from build123d import *

# Parameters (mm, degrees)
SKETCH004_W   = 113.720292
SKETCH004_H   = 7.903844
SKETCH004_R   = 1.75
SKETCH004_R_2 = 1.5
PAD_DEPTH     = 1


with BuildPart() as part:
    # Sketch004 → Pad (new body)
    with BuildSketch(Plane.XY):
        Rectangle(SKETCH004_W, SKETCH004_H)
        with Locations((-52.5, 0)):
            Circle(SKETCH004_R, mode=Mode.SUBTRACT)
        with Locations((52.5, 0)):
            Circle(SKETCH004_R, mode=Mode.SUBTRACT)
        Circle(SKETCH004_R_2, mode=Mode.SUBTRACT)
    extrude(amount=PAD_DEPTH)


solid = part.part
Verification items for the finished model (mm, model axes). Coordinates: 2 decimals unless noted, no trailing zeros. Order: outer loops, then holes, each group sorted by start corner. A loop starts at its lowest first (then second) coordinate and runs counter-clockwise, first axis right, second up. Notation, with made-up numbers: (-4.5, -14) -> (49.5, -14) arc R30 cw to (49.5, 12) -> close; hole circle Ø2 at (85.5, 63.5). An arc over 180 degrees is marked (long way). Put each result on its own line as item: value. Start each with the question number.
1. Material ranges on L1, parallel to Y at x = -52.5, z = 0.3; L2, parallel to Y at x = 1, z = 0.1, recorded low to high. Write a range as [from, to].
2. Go/stop test with flat-tipped pins: pin 1 Ø2 at (x, y) = (52.5, 0) entering from +Z; pin 2 Ø4 at (x, y) = (0, -1.5) entering from -Z. Record where each tip stops, or that it passes through.
3. Cross-section at C-C, the plane z = 0.85. Record the boundary of the cut face in (x, y), then the cut area to 3 significant figures.
4. Mould release check, pull along Y, two halves, no side actions. Record for faces 1 (the flat face through (-1, 2, 0)), 2 (the cylindrical face through (54.117, -0.67, 0.493)): released by +Y, released by -Y, zero draft, split by the parting line, or undercut.
5. Cross-section at B-B, the plane x = 52.5. Record the boundary of the cut face in (y, z).
6. Cross-section at D-D, the plane x = 0. Record the boundary of the cut face in (y, z).
7. Cross-section at A-A, the plane y = 0. Record the boundary of the cut face in (x, z), then the cut area to 3 significant figures.
Computed:
1. L1: [-3.95, -1.75], [1.75, 3.95]
1. L2: [-3.95, -1.12], [1.12, 3.95]
2. pin 1: through
2. pin 2: z = 0
3. outline: (-56.86, -3.95) -> (56.86, -3.95) -> (56.86, 3.95) -> (-56.86, 3.95) -> close; hole circle Ø3.5 at (-52.5, 0); hole circle Ø3 at (0, 0); hole circle Ø3.5 at (52.5, 0)
3. area: 873 mm2
4. face 1: zero draft
4. face 2: undercut
5. outline: (-3.95, 0) -> (-1.75, 0) -> (-1.75, 1) -> (-3.95, 1) -> close; (1.75, 0) -> (3.95, 0) -> (3.95, 1) -> (1.75, 1) -> close
6. outline: (-3.95, 0) -> (-1.5, 0) -> (-1.5, 1) -> (-3.95, 1) -> close; (1.5, 0) -> (3.95, 0) -> (3.95, 1) -> (1.5, 1) -> close
7. outline: (-56.86, 0) -> (-54.25, 0) -> (-54.25, 1) -> (-56.86, 1) -> close; (-50.75, 0) -> (-1.5, 0) -> (-1.5, 1) -> (-50.75, 1) -> close; (1.5, 0) -> (50.75, 0) -> (50.75, 1) -> (1.5, 1) -> close; (54.25, 0) -> (56.86, 0) -> (56.86, 1) -> (54.25, 1) -> close
7. area: 104 mm2
